from build123d import *

# Parameters (mm, degrees)
SKETCH2_W               = 200.4
SKETCH2_H               = 153.4
SKETCH2_W_2             = 150.4
SKETCH2_H_2             = 20.4
BOSS_EXTRUDE1_DEPTH     = 10
CUT_EXTRUDE1_REACH      = 234.876
SKETCH4_R               = 5
CUT_EXTRUDE2_DEPTH      = 157.241095746
CUT_EXTRUDE2_DEPTH_BACK = 157.241095746
SKETCH7_W               = 25
SKETCH7_H               = 25
SKETCH8_W               = 200.4
SKETCH8_H               = 11
CUT_EXTRUDE3_DEPTH      = 10


with BuildPart() as part:
    # Sketch2 → Boss-Extrude1 (new, symmetric)
    with BuildSketch(Plane.XY):
        with Locations((0, 41.5)):
            Rectangle(SKETCH2_W, SKETCH2_H)
        Rectangle(SKETCH2_W_2, SKETCH2_H_2, mode=Mode.SUBTRACT)
    extrude(amount=BOSS_EXTRUDE1_DEPTH, both=True)

    # Sketch4 → Cut-Extrude1 (cut, up to next)
    with BuildSketch(Plane(origin=(100.2, 0, 0), x_dir=(0, 0, -1), z_dir=(1, 0, 0)), mode=Mode.PRIVATE) as cut_extrude1_sk1:
        Circle(SKETCH4_R)
    cut_extrude1_tool1 = extrude(cut_extrude1_sk1.sketch, amount=-CUT_EXTRUDE1_REACH, mode=Mode.PRIVATE) & part.part
    add(cut_extrude1_tool1.solids().sort_by_distance((100.2, 0, 0))[0], mode=Mode.SUBTRACT)

    # Sketch7 → Cut-Extrude2 (cut, two sides: drawn at the far end of the back side and taken through both)
    with BuildSketch(Plane.XY.offset(10).offset(-CUT_EXTRUDE2_DEPTH_BACK)):
        with Locations((0, 85.2)):
            Rectangle(SKETCH7_W, SKETCH7_H)
    extrude(amount=CUT_EXTRUDE2_DEPTH + CUT_EXTRUDE2_DEPTH_BACK, mode=Mode.SUBTRACT)

    # Sketch8 → Cut-Extrude3 (cut)
    with BuildSketch(Plane(origin=(0, 118.2, 0), x_dir=(1, 0, 0), z_dir=(0, 1, 0))):
        with Locations((0, -4.5)):
            Rectangle(SKETCH8_W, SKETCH8_H)
    extrude(amount=-CUT_EXTRUDE3_DEPTH, mode=Mode.SUBTRACT)


solid = part.part
CAD build for the part. Positions are in the model's coordinates, mm. A direction names the side the tool comes from. Coordinates: 2 decimals unless noted, no trailing zeros. Loops run counter-clockwise (first coordinate to the right, second up) from the corner with the lowest first, then second, coordinate; pieces in that order, holes last. Notation, with made-up numbers: (22, -4) - (28, -4) arc R12 ccw to (28, 5) - close; hole circle Ø10 at (64.5, -12). An arc over 180 degrees is marked (long way). Use one line per item in the form item = value. Start each with the question number.
1) Band-saw the part on B-B (x = 27). Give the cut face in (y, z), and give its area (3 significant figures).
2) Two-plate mould, pull along X, no slides. Class faces 1 (the face through (-100.2, 40, 0)), 2 (the face through (-1, 43, -10)), 3 (the face through (-1, 10.2, 0)): +X half, -X half, draft (parallel to the pull), parting line (faces both ways), or undercut.
3) Flat gauge pin, fed straight in: pin 1 (5.5 mm diameter, centred on x = -21.5, z = 5, fed in from +Y). Where does the tip first touch, or does it go through?
4) Band-saw the part on A-A (y = 0). Give the cut face in (x, z).
5) Drill centre lines: L1, parallel to Y at x = -50.5, z = -0.75; L2, parallel to Y at x = 82, z = 0; L3, parallel to X at y = -3, z = -6.75. Where is each one in solid material? Low to high. Write a range as from..to.
6) Tool access for faces 4 (the face through (-1, 108.2, 4)), 5 (the face through (0, 97.7, 0)), 6 (the face through (100.2, 40, 0)), 7 (the face through (87.88, -4.88, 1.08)): list every direction of +Z, -Z, +X, -X, +Y, -Y with a clear straight run to the whole face (end or side of a thin tool).
7) Band-saw the part on C-C (x = 82). Give the cut face in (y, z), and give its area (3 significant figures).
Check values:
q1.outline = (-35.2, -10) - (-10.2, -10) - (-10.2, 10) - (-35.2, 10) - close; (10.2, -10) - (118.2, -10) - (118.2, -1) - (108.2, -1) - (108.2, 10) - (10.2, 10) - close
q1.area = 2,550 mm2
q2.face_1 = -X half
q2.face_2 = draft
q2.face_3 = undercut
q3.pin_1 = 108.2
q4.outline = (-100.2, -10) - (-75.2, -10) - (-75.2, 10) - (-100.2, 10) - close; (75.2, -10) - (100.2, -10) - (100.2, -5) - (75.2, -5) - close; (75.2, 5) - (100.2, 5) - (100.2, 10) - (75.2, 10) - close
q5.L1 = -35.2..-10.2, 10.2..108.2
q5.L2 = -35.2..-5, 5..108.2
q5.L3 = -100.2..-75.2, 75.2..100.2
q6.face_4 = +Z, +X, -X, +Y
q6.face_5 = +Z, -Z
q6.face_6 = +Z, -Z, +X, +Y, -Y
q6.face_7 = +X
q7.outline = (-35.2, -10) - (118.2, -10) - (118.2, -1) - (108.2, -1) - (108.2, 10) - (-35.2, 10) - close; hole circle Ø10 at (0, 0)
q7.area = 2,880 mm2
